from build123d import *

# Parameters (mm, degrees)
SKETCH21_R           = 1.7
SKETCH21_W           = 26.12
SKETCH21_H           = 8
BOSS_EXTRUDE18_DEPTH = 6
SKETCH22_W           = 5
SKETCH22_H           = 32.12
BOSS_EXTRUDE19_DEPTH = 5


with BuildPart() as part:
    # Sketch21 → Boss-Extrude18 (new body)
    with BuildSketch(Plane(origin=(0, 0, 0), x_dir=(1, 0, 0), z_dir=(0, 1, 0))):
        Polygon((0, 73), (-16.06, 73), (-16.06, 16.06), (-73, 16.06), (-73, 0), (-73, -16.06), (-16.06, -16.06), (-16.06, -73), (0, -73), (16.06, -73), (16.06, -16.06), (73, -16.06), (73, 0), (73, 16.06), (16.06, 16.06), (16.06, 73), align=None)
        with Locations(Location((-12.56, 31.04, 0), (0, 0, 270))):
            Circle(SKETCH21_R, mode=Mode.SUBTRACT)
        with Locations(Location((12.56, 31.04, 0), (0, 0, 270))):
            Circle(SKETCH21_R, mode=Mode.SUBTRACT)
        with Locations((0, 20.6)):
            Rectangle(SKETCH21_W, SKETCH21_H, mode=Mode.SUBTRACT)
    extrude(amount=BOSS_EXTRUDE18_DEPTH)

    # Sketch22 → Boss-Extrude19 (add)
    with BuildSketch(Plane(origin=(0, 6, 0), x_dir=(1, 0, 0), z_dir=(0, 1, 0))):
        with Locations((-70.5, 0)):
            Rectangle(SKETCH22_W, SKETCH22_H)
    extrude(amount=BOSS_EXTRUDE19_DEPTH)


solid = part.part
Here's how the part is built. I have some questions about the finished solid (model axes, mm). A direction names the side the tool comes from. Coordinates: 2 decimals unless noted, no trailing zeros. Write each loop counter-clockwise with the first axis right and the second up, starting at its lowest first coordinate (ties: lowest second). Pieces come first, ordered by that corner, then holes.
Item 1: I want a section at C-C on z = -2. Write out the boundary of the cut face in (x, y).
Item 2: Will these pins go through, and if not, where does the flat tip stop? pin 1 (3 mm diameter, centred on x = -6.5, z = 36, fed in from +Y); pin 2 (1.8 mm diameter, centred on y = 4, z = 43, fed in from -X); pin 3 (6.5 mm diameter, centred on y = 1.5, z = -22, fed in from +X); pin 4 (8 mm diameter, centred on x = -42.5, z = -2.5, fed in from -Y).
Item 3: I want a section at A-A on z = -31.04. Write out the boundary of the cut face in (x, y), and give its area (3 significant figures).
Item 4: I want a section at D-D on x = -48.5. Write out the boundary of the cut face in (y, z), and give its area (3 significant figures).
Item 5: On a 3-axis mill with a long thin cutter (end or side, diameter ignored), from which of +Z, -Z, +X, -X, +Y, -Y can I reach the whole of each face in a straight line? I mean faces 1 (the flat face through (16.06, 3, 45)), 2 (the flat face through (-68, 8, 0)), 3 (the flat face through (-16.06, 3, 44)). Say none if no direction works.
Item 6: If we mould it in two halves opening along Z, with no side actions, what happens to faces 4 (the flat face through (0, 3, 73)), 5 (the flat face through (-13.06, 3, -21)), 6 (the flat face through (0, 3, -73)), 7 (the flat face through (0, 3, -24.6))? For each: +Z half, -Z half, draft (parallel to the pull), parting line (faces both ways), or undercut.
Item 7: If I drill on line 1 (X direction, y = 4.25, z = -31.04); line 2 (Z direction, x = 4.5, y = 5.5); line 3 (X direction, y = 9.75, z = 6.5), over which ranges is the centre line in solid material (lowest first)?
Item 8: I want a section at B-B on y = 4.25. Write out the boundary of the cut face in (x, z).
Findings below:
1. outline: (-73, 0) - (73, 0) - (73, 6) - (-68, 6) - (-68, 11) - (-73, 11) - close
2. pin 1: stops at y = 6
2. pin 2: stops at x = -16.06
2. pin 3: stops at x = 16.06
2. pin 4: stops at y = 0
3. outline: (-16.06, 0) - (-14.26, 0) - (-14.26, 6) - (-16.06, 6) - close; (-10.86, 0) - (10.86, 0) - (10.86, 6) - (-10.86, 6) - close; (14.26, 0) - (16.06, 0) - (16.06, 6) - (14.26, 6) - close
3. area: 152 mm2
4. outline: (0, -16.06) - (6, -16.06) - (6, 16.06) - (0, 16.06) - close
4. area: 193 mm2
5. face 1: +Z, +X, +Y, -Y
5. face 2: +Z, -Z, +X, +Y
5. face 3: +Z, -X, +Y, -Y
6. face 4: +Z half
6. face 5: undercut
6. face 6: -Z half
6. face 7: undercut
7. line 1: x = -16.06 to -14.26, -10.86 to 10.86, 14.26 to 16.06
7. line 2: z = -73 to -24.6, -16.6 to 73
7. line 3: x = -73 to -68
8. outline: (-73, -16.06) - (-16.06, -16.06) - (-16.06, -73) - (16.06, -73) - (16.06, -16.06) - (73, -16.06) - (73, 16.06) - (16.06, 16.06) - (16.06, 73) - (-16.06, 73) - (-16.06, 16.06) - (-73, 16.06) - close; hole circle Ø3.4 at (-12.56, -31.04); hole (-13.06, -24.6) - (13.06, -24.6) - (13.06, -16.6) - (-13.06, -16.6) - close; hole circle Ø3.4 at (12.56, -31.04)
